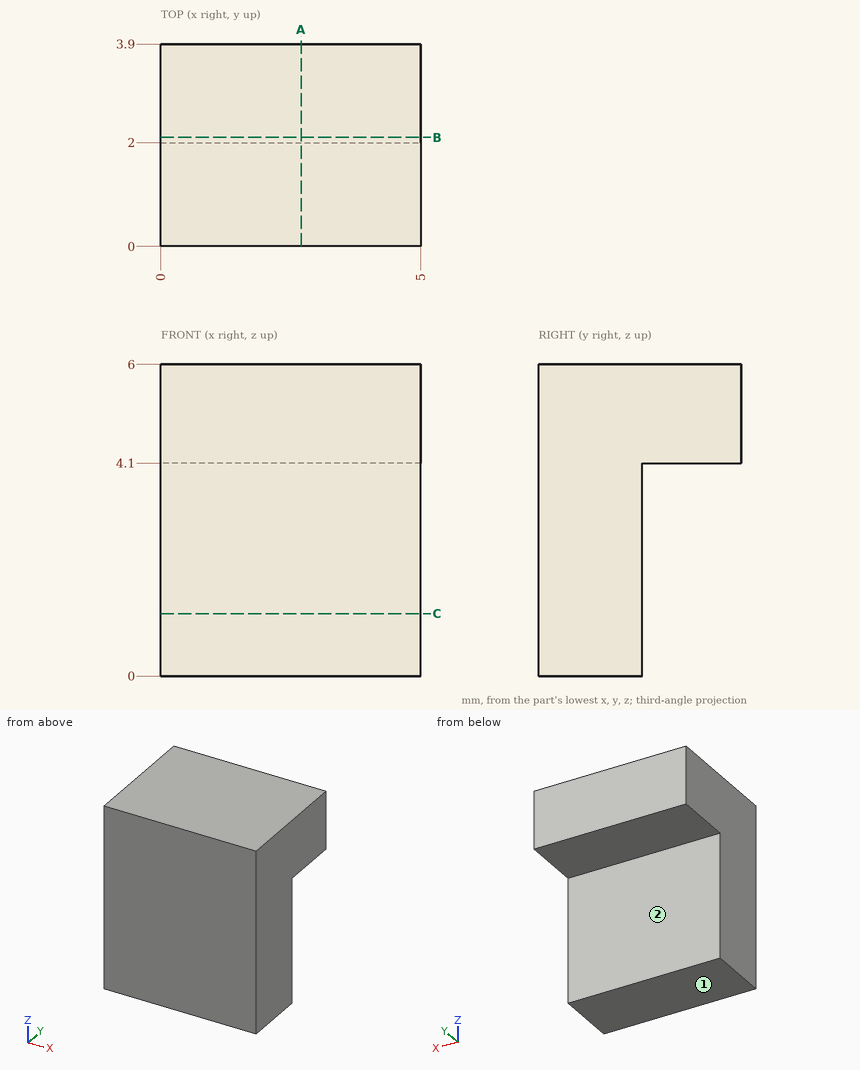
Source: three-view drawing plus pictorial views. Frame: mm from the lowest corner of the part. A direction names the side the tool comes from. Round coordinates to 2 decimals unless told otherwise and drop trailing zeros. Loops run counter-clockwise (first coordinate to the right, second up) from the corner with the lowest first, then second, coordinate; pieces in that order, holes last.
Q1. Section C-C on z = 1.2. Return loops of the section in (x, y).
Q2. Material intervals for L1, parallel to Z at x = 4.4, y = 2.55; L2, parallel to Y at x = 2.3, z = 3.9, sorted ascending.
Q3. Section B-B on y = 2.1. Return loops of the section in (x, z).
Q4. Pin query (flat end, axial travel): P1, Ø2, axis at x = 2.5, z = 1, coming from the +Y side. Return the tip coordinate at first contact, or that it passes through.
Q5. Access query for the marked faces 1 and 2. Directions: +Z, -Z, +X, -X, +Y, -Y. A direction counts if a zero-diameter tool reaches every point of the face in a straight line with its end or side. Return the directions, or none.
Q6. Section A-A on x = 2.7. Return loops of the section in (y, z).
Evaluation:
1. outline: (0, 0) - (5, 0) - (5, 2) - (0, 2) - close
2. L1: z = 4.1 to 6
2. L2: y = 0 to 2
3. outline: (0, 4.1) - (5, 4.1) - (5, 6) - (0, 6) - close
4. P1: stops at y = 2
5. face 1: -Z, +X, -X, +Y, -Y
5. face 2: -Z, +X, -X, +Y
6. outline: (0, 0) - (2, 0) - (2, 4.1) - (3.9, 4.1) - (3.9, 6) - (0, 6) - close
